Work out the finished part from the listing and answer in its coordinate system (mm). A direction names the side the tool comes from. Give positions to 0.01 mm unless a question says otherwise; leave off trailing zeros. One line per question, with ' | ' between items. Start each with the question number.
1. For a pull along Y with two mould halves and no side action, classify faces 4 (the face through (11.207, -3.529, -11.84)), 5 (the face through (27.605, 3.639, -26.224)), 6 (the face through (35, -9, -31)) as released by +Y, released by -Y, zero draft, split by the parting line, or undercut.
2. Find the intervals of material crossed by line 1 (Y direction, x = 10, z = -32.5); line 2 (Z direction, x = 23.75, y = 0); line 3 (X direction, y = -6.75, z = -8), in increasing order.
3. Each of these flat-tipped pins is pushed along its axis until it touches: pin 1 (4 mm diameter, centred on y = 4.5, z = -19.5, fed in from -X); pin 2 (5 mm diameter, centred on x = -5.5, y = 1, fed in from -Z); pin 3 (11.5 mm diameter, centred on y = 0, z = -35, fed in from +X). Where does it stop, or does it pass through?
4. Which of the six approach directions +Z, -Z, +X, -X, +Y, -Y give full straight-line access (tool end or side, diameter ignored) to faces 1 (the face through (4.38, 8.43, -7.6)), 2 (the face through (23.25, -0.52, -46.74)), 3 (the face through (-4, 9, 0))?
from build123d import *

# Parameters (mm, degrees)
SKETCH2_R          = 11.75
SKETCH2_R_2        = 9.5
SKETCH40_OUTSIDE_W = 63.83
SKETCH40_OUTSIDE_H = 40.58
SKETCH40_OUTSIDE_R = 11.45
CUT_EXTRUDE2_DEPTH = 15
CUT_EXTRUDE2_TAPER = 2
SKETCH41_OUTSIDE_W = 63.83
SKETCH41_OUTSIDE_H = 40.58
SKETCH41_OUTSIDE_R = 11.45
CUT_EXTRUDE3_DEPTH = 15
CUT_EXTRUDE3_TAPER = 2


with BuildPart() as part:
    # Sweep1: sweep along a path in Sketch1
    with BuildLine(Plane(origin=(0, 0, 0), x_dir=(1, 0, 0), z_dir=(0, 1, 0))) as sweep1_path:
        Line((0, 0), (0, 15))
        ThreePointArc((0, 15), (5.857864376, 29.142135624), (20, 35))
        Line((20, 35), (35, 35))
    # Sketch2 → Sweep1 (sweep)
    with BuildSketch(Plane.XY):
        Circle(SKETCH2_R)
        Circle(SKETCH2_R_2, mode=Mode.SUBTRACT)
    sweep(path=sweep1_path.line)

    # Sketch40 outside → Cut-Extrude2 (cut)
    with BuildSketch(Plane.XY):
        with Locations((11.625, 0)):
            Rectangle(SKETCH40_OUTSIDE_W, SKETCH40_OUTSIDE_H)
        Circle(SKETCH40_OUTSIDE_R, mode=Mode.SUBTRACT)
    extrude(amount=-CUT_EXTRUDE2_DEPTH, taper=CUT_EXTRUDE2_TAPER, mode=Mode.SUBTRACT)

    # Sketch41 outside → Cut-Extrude3 (cut)
    with BuildSketch(Plane(origin=(35, 0, 0), x_dir=(0, 0, -1), z_dir=(1, 0, 0))):
        with Locations((23.375, 0)):
            Rectangle(SKETCH41_OUTSIDE_W, SKETCH41_OUTSIDE_H)
        with Locations((35, 0)):
            Circle(SKETCH41_OUTSIDE_R, mode=Mode.SUBTRACT)
    extrude(amount=-CUT_EXTRUDE3_DEPTH, taper=CUT_EXTRUDE3_TAPER, mode=Mode.SUBTRACT)


solid = part.part
Conclusion:
1) face 4: split by the parting line | face 5: undercut | face 6: zero draft
2) line 1: -11.75 to -9.5, 9.5 to 11.75 | line 2: -46.75 to -44.5, -25.5 to -23.25 | line 3: -9.59 to -6.68, 6.68 to 9.59
3) pin 1: x = -11.23 | pin 2: z = -36.84 | pin 3: x = 5.61
4) face 1: +Z | face 2: +X | face 3: +Z, +X, -X, +Y, -Y
